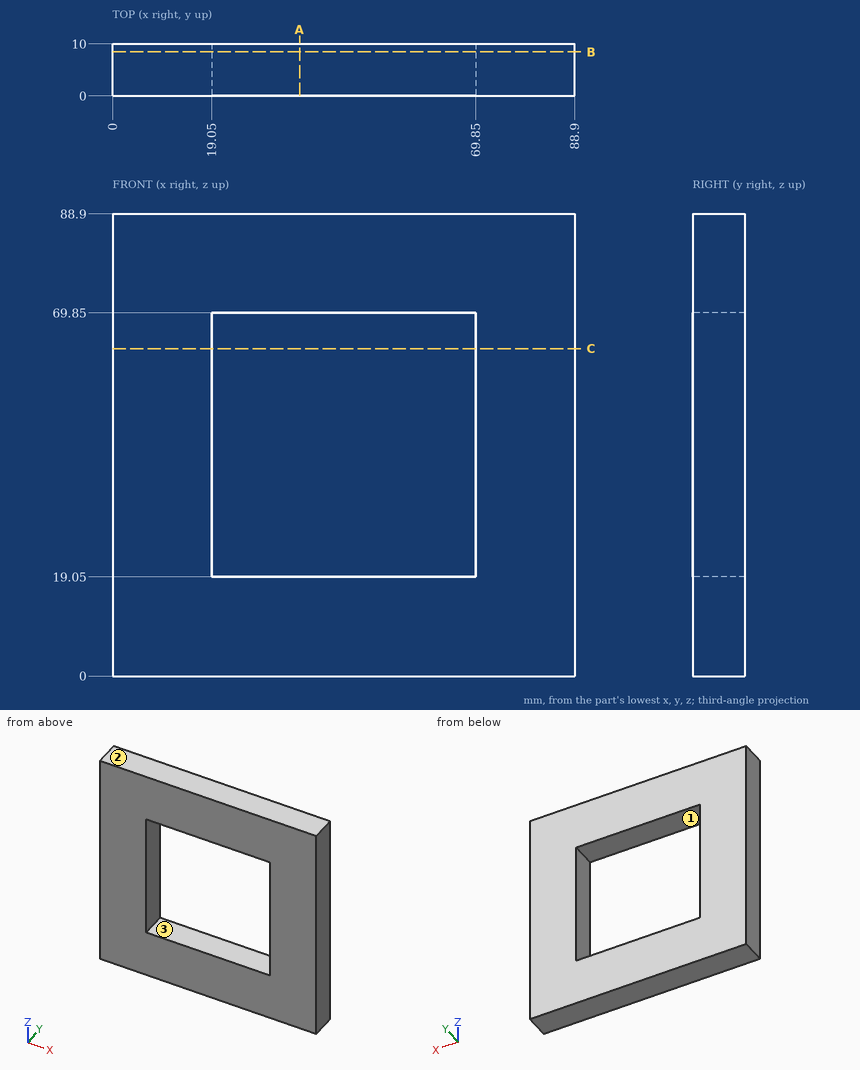
Can you work these out from the drawing? Everything is in mm from the part's minimum corner. Give positions to 0.01 mm unless a question says otherwise; leave off trailing zeros. Order: outer loops, then holes, each group sorted by start corner. A loop starts at its lowest first (then second) coordinate and runs counter-clockwise, first axis right, second up.
1. Suppose I cut it at C-C (z = 63). List the corners of the cut face in (x, y) for me.
2. We'd pull the mould along X, two halves only. Please class the marked faces 1, 2 and 3: pulls with the +X half, pulls with the -X half, needs draft (parallel to the pull), parting line crosses it, or undercut.
3. Suppose I cut it at A-A (x = 36). List the corners of the cut face in (y, z) for me.
4. Suppose I cut it at B-B (y = 8.5). List the corners of the cut face in (x, z) for me, plus the area to 3 significant figures.
5. I need wall thicknesses on L1, parallel to Z at x = 21, y = 8.5. Which ranges of the line are inside material? Lowest first, please.
Solved:
1. outline: (0, 0) - (19.05, 0) - (19.05, 10) - (0, 10) - close; (69.85, 0) - (88.9, 0) - (88.9, 10) - (69.85, 10) - close
2. face 1: undercut
2. face 2: needs draft
2. face 3: undercut
3. outline: (0, 0) - (10, 0) - (10, 19.05) - (0, 19.05) - close; (0, 69.85) - (10, 69.85) - (10, 88.9) - (0, 88.9) - close
4. outline: (0, 0) - (88.9, 0) - (88.9, 88.9) - (0, 88.9) - close; hole (19.05, 19.05) - (69.85, 19.05) - (69.85, 69.85) - (19.05, 69.85) - close
4. area: 5,320 mm2
5. L1: z = 0 to 19.05, 69.85 to 88.9
